Design review of the part built by this model. Coordinates are the model's own, in mm. Face numbers are marked on the shaded views. A direction names the side the tool comes from. Coordinates: 2 decimals unless noted, no trailing zeros. Write each loop counter-clockwise with the first axis right and the second up, starting at its lowest first coordinate (ties: lowest second). Pieces come first, ordered by that corner, then holes.
Q1. For L1, parallel to Z at x = 0, y = 1.8; L2, parallel to X at y = 4.75, z = 15; L3, parallel to Y at x = 5, z = 18.5, list the stretches that pass through material, from the lowest coordinate up.
Q2. Take a section at B-B, the plane z = 0. Write out the cut boundary in (x, y), plus the area to 3 significant figures.
Q3. For pin 1 Ø1 at (y, z) = (3, 2.5) entering from +X; pin 2 Ø2 at (y, z) = (1, 0) entering from +X; pin 3 Ø3 at (x, y) = (-3.5, 1) entering from -Z, all flat-tipped, find the tip position at first contact; note any pin that passes through.
Q4. For the marked faces 4 and 5, list the 3-axis set-ups (+Z, -Z, +X, -X, +Y, -Y) from which the entire face can be reached by the end or side of a thin tool; tool diameter is ignored.
Q5. Take a section at D-D, the plane y = 2.4. Write out the cut boundary in (x, z), plus the area to 3 significant figures.
Q6. The part is to be moulded in two halves that separate along X. For the marked faces 1, 2 and 3, say which applies: released by +X, released by -X, zero draft, split by the parting line, or undercut.
Q7. Take a section at A-A, the plane x = 0. Write out the cut boundary in (y, z), plus the area to 3 significant figures.
Q8. Take a section at C-C, the plane x = -8. Write out the cut boundary in (y, z), plus the area to 3 significant figures.
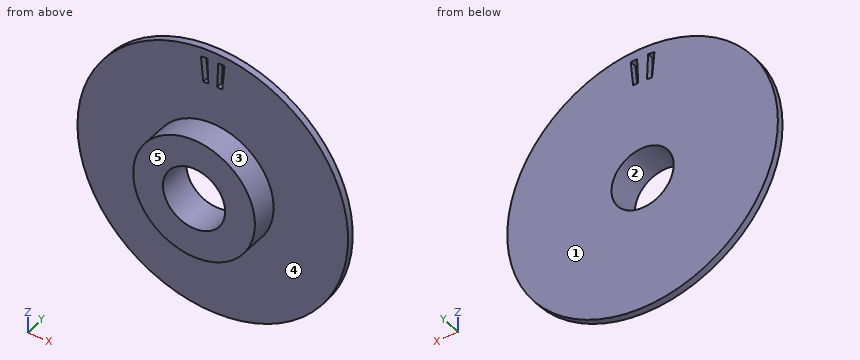
Autodesk Inventor part; units mm, degrees
ref_plane "YZ Plane" through (0, 0, 0) normal (1, 0, 0) x (0, 1, 0)
ref_plane "XZ Plane" through (0, 0, 0) normal (0, 1, 0) x (-1, 0, 0)
ref_plane "XY Plane" through (0, 0, 0) normal (0, 0, 1) x (1, 0, 0)
sketch "Sketch1" plane through (0, 0, 0) normal (0, 1, 0) x (-1, 0, 0)
  circle A0 centre (0, 0) radius 20
  line L0 (0, 0) -> (20, 0)
  circle A1 centre (0, 0) radius 4.6
  dimension "d1" = 40
  dimension "d6" = 9.2
extrude "Extrusion1" add sketch "Sketch1" along normal blind 5
sketch "Sketch2" plane through (0, 0, 0) normal (0, -1, 0) x (1, 0, 0)
  circle A0 centre (0, 0) radius 4.6
  circle A1 centre (0, 0) radius 20
  circle A2 centre (0, 0) radius 9
  circle A3 centre (0, 0) radius 20
  dimension "d7" = 18
extrude "Extrusion2" cut sketch "Sketch2" against normal blind 4 contours A1
sketch "Sketch3" plane through (0, 5, 0) normal (0, 1, 0) x (1, 0, 0)
  circle A0 centre (0, 0) radius 4.6
  circle A1 centre (0, 0) radius 20
  line L0 (0, 0) -> (0, -20)
  circle A2 centre (0, 0) radius 20
  line L1 (2.4, -13.5) -> (2.4, -20)
  line L2 (2.4, -20) -> (-2.4, -20)
  line L3 (-2.4, -20) -> (-2.4, -13.5)
  line L4 (-2.4, -13.5) -> (2.4, -13.5)
  line L5 (2.4, -13.5) -> (-2.4, -20) construction
  line L6 (2.4, -20) -> (-2.4, -13.5) construction
  line L7 (0.25, -18.6) -> (1.75, -18.6)
  line L8 (1.75, -18.6) -> (1.75, -14.9)
  line L9 (1.75, -14.9) -> (0.25, -14.9)
  line L10 (0.25, -14.9) -> (0.25, -18.6)
  line L11 (-0.25, -18.6) -> (-1.75, -18.6)
  line L12 (-1.75, -18.6) -> (-1.75, -14.9)
  line L13 (-1.75, -14.9) -> (-0.25, -14.9)
  line L14 (-0.25, -14.9) -> (-0.25, -18.6)
  arc A3 (-0.8149, -18.6644) -> (-1.75, -18.6) centre (0, 0) ccw
  arc A4 (-0.65, -14.8879) -> (-1.3959, -14.8366) centre (0, 0) ccw
  line L15 (0, 0) -> (-0.65, -14.8879)
  line L16 (0, 0) -> (0.65, -14.8879)
  line L17 (0, 0) -> (-1.3959, -14.8366)
  line L18 (0, 0) -> (1.3959, -14.8366)
  arc A5 (-1.3959, -14.8366) -> (-0.65, -14.8879) centre (0, 0) ccw
  arc A6 (-1.3886, -18.6305) -> (-0.8149, -18.6644) centre (0, 0) ccw
  arc A7 (-1.75, -18.6) -> (-1.3886, -18.6305) centre (0, 0) ccw
  line L19 (-0.65, -14.8879) -> (-0.8149, -18.6644)
  line L20 (-1.3959, -14.8366) -> (-1.75, -18.6)
  line L21 (1.3959, -14.8366) -> (1.75, -18.6)
  line L22 (0.65, -14.8879) -> (0.8149, -18.6644)
  point P0 (0, -16.75)
  dimension "d10" = 0
  dimension "d11" = 4.8
  dimension "d12" = 6.5
  dimension "d13" = 1.5
  dimension "d14" = 3.7
  dimension "d17" = 1.4
  dimension "d40" = 2
  dimension "d41" = 0.25
  dimension "d76" = 5
  dimension "d77" = 2.5
extrude "Extrusion4" cut sketch "Sketch3" against normal blind 10 contours A5 L19 L13 L20 | L21 L9 L22 A4 | L13 L19 L11 L20 | L21 L7 L22 L9 | L11 L19 A6 A7 | A3 L22 L7
equation "\"d17\" = -0.5 * d14 + 0.5 * d12"
equation "\"d41\" = -0.5 * d13 + 0.5 * d40"
equation "\"d77\" = 0.5 * d76"
properties part number "BigPositionDisk"
Responses:
1. L1: z = -9 to -4.6, 4.6 to 9
1. L2: x = -13.23 to -1.41, -0.65 to 0.65, 1.41 to 13.23
1. L3: y = 4 to 5
2. outline: (-20, 4) - (-9, 4) - (-9, 0) - (-4.6, 0) - (-4.6, 5) - (-20, 5) - close; (4.6, 0) - (9, 0) - (9, 4) - (20, 4) - (20, 5) - (4.6, 5) - close
2. area: 66.0 mm2
3. pin 1: stops at x = 8.77
3. pin 2: stops at x = 9
3. pin 3: stops at z = -8.77
4. face 4: -Y
4. face 5: +Z, -Z, +X, -X, -Y
5. outline: circle Ø18 at (0, 0); hole circle Ø9.2 at (0, 0)
5. area: 188 mm2
6. face 1: zero draft
6. face 2: undercut
6. face 3: split by the parting line
7. outline: (0, -9) - (4, -9) - (4, -20) - (5, -20) - (5, -4.6) - (0, -4.6) - close; (0, 4.6) - (5, 4.6) - (5, 20) - (4, 20) - (4, 9) - (0, 9) - close
7. area: 66.0 mm2
8. outline: (0, -4.12) - (4, -4.12) - (4, -18.33) - (5, -18.33) - (5, 18.33) - (4, 18.33) - (4, 4.12) - (0, 4.12) - close
8. area: 69.6 mm2
